```python
from build123d import *

# Parameters (mm, degrees)
F0_W          = 100.84
F0_H          = 99.31
F0_R          = 1.5
F0_R_2        = 2
F1_DEPTH      = 2
F3_W          = 15
F3_H          = 10
F3_W_2        = 41
F3_H_2        = 20.5
F4_DEPTH      = 13
F4_DEPTH_BACK = 2
F5_W          = 18
F5_H          = 35.5
F6_DEPTH      = 17
F8_W          = 8
F8_H          = 3
F9_DEPTH      = 2


with BuildPart() as f1:
    # F0 (on Top) → F1 (new body)
    with BuildSketch(Plane.XY):
        Rectangle(F0_W, F0_H)
        with Locations((-47.88, -46.865)):
            Circle(F0_R, mode=Mode.SUBTRACT)
        with Locations((-42.29, -44.825)):
            Circle(F0_R_2, mode=Mode.SUBTRACT)
        with Locations((-42.29, -36.445)):
            Circle(F0_R_2, mode=Mode.SUBTRACT)
        with Locations((-42.29, -24.765)):
            Circle(F0_R_2, mode=Mode.SUBTRACT)
        with Locations((-42.29, -16.635)):
            Circle(F0_R_2, mode=Mode.SUBTRACT)
        with Locations((-42.29, -4.955)):
            Circle(F0_R_2, mode=Mode.SUBTRACT)
        with Locations((42.29, -44.825)):
            Circle(F0_R_2, mode=Mode.SUBTRACT)
        with Locations((47.88, -46.865)):
            Circle(F0_R, mode=Mode.SUBTRACT)
        with Locations((42.29, -36.445)):
            Circle(F0_R_2, mode=Mode.SUBTRACT)
        with Locations((42.29, -24.765)):
            Circle(F0_R_2, mode=Mode.SUBTRACT)
        with Locations((42.29, -16.635)):
            Circle(F0_R_2, mode=Mode.SUBTRACT)
        with Locations((42.29, -4.955)):
            Circle(F0_R_2, mode=Mode.SUBTRACT)
        with Locations((-42.29, 3.175)):
            Circle(F0_R_2, mode=Mode.SUBTRACT)
        with Locations((-42.29, 14.855)):
            Circle(F0_R_2, mode=Mode.SUBTRACT)
        with Locations((-42.29, 22.985)):
            Circle(F0_R_2, mode=Mode.SUBTRACT)
        with Locations((-48.06, 25.525)):
            Circle(F0_R, mode=Mode.SUBTRACT)
        with Locations((42.29, 3.175)):
            Circle(F0_R_2, mode=Mode.SUBTRACT)
        with Locations((42.29, 14.855)):
            Circle(F0_R_2, mode=Mode.SUBTRACT)
        with Locations((42.29, 22.985)):
            Circle(F0_R_2, mode=Mode.SUBTRACT)
        with Locations((47.88, 25.275)):
            Circle(F0_R, mode=Mode.SUBTRACT)
    extrude(amount=F1_DEPTH)

    # F3 (on offset) → F4 (join, two sides)
    with BuildSketch(Plane.XY.offset(2)) as f4_sk:
        with Locations((-38.09, 54.655)):
            Rectangle(F3_W, F3_H)
        with Locations((23.92, 59.905)):
            Rectangle(F3_W_2, F3_H_2)
    extrude(amount=F4_DEPTH)
    extrude(f4_sk.sketch, amount=-F4_DEPTH_BACK)

    # F5 (on offset) → F6 (join)
    with BuildSketch(Plane.XY.offset(2)):
        with Locations((0, -31.905)):
            Rectangle(F5_W, F5_H)
    extrude(amount=F6_DEPTH)

    # F8 (on offset) → F9 (join)
    with BuildSketch(Plane.XZ.offset(49.655)):
        with Locations((0, 17.5)):
            Rectangle(F8_W, F8_H)
    extrude(amount=F9_DEPTH)


solid = f1.part
```
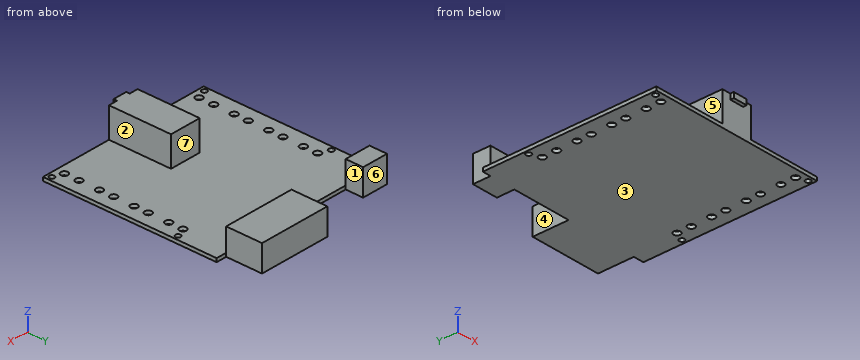
Geometry: final body of the model. Coordinates: model frame, mm. Face numbers are marked on the shaded views. A direction names the side the tool comes from. Give positions to 0.01 mm unless a question says otherwise; leave off trailing zeros. Loops run counter-clockwise (first coordinate to the right, second up) from the corner with the lowest first, then second, coordinate; pieces in that order, holes last. Notation, with made-up numbers: (-16, 26) -> (20, 26) arc R8 ccw to (20, 35) -> close; hole circle Ø10 at (-9.75, 57). An arc over 180 degrees is marked (long way). Use one line per item in the form item = value.
Item 1: Draft query along X for the marked faces 1, 2 and 3. Return one class per face: pulls with the +X half, pulls with the -X half, needs draft (parallel to the pull), parting line crosses it, or undercut.
A:
face_1 = undercut
face_2 = pulls with the +X half
face_3 = needs draft
Item 2: Access query for the marked faces 4, 5, 6 and 7. Directions: +Z, -Z, +X, -X, +Y, -Y. A direction counts if a zero-diameter tool reaches every point of the face in a straight line with its end or side. Return the directions, or none.
A:
face_4 = +Z, -Z, +Y
face_5 = +Z, -X, +Y, -Y
face_6 = +Z, -Z, -X, +Y
face_7 = +Z, +X, -X
Item 3: Section query A-A on z = 12.5. Output: boundary loops of the cut face in (x, y) (3 decimals), and give its area (3 significant figures).
A:
outline = (-45.59, 49.655) -> (-30.59, 49.655) -> (-30.59, 59.655) -> (-45.59, 59.655) -> close; (-9, -49.655) -> (9, -49.655) -> (9, -14.155) -> (-9, -14.155) -> close; (3.42, 49.655) -> (44.42, 49.655) -> (44.42, 70.155) -> (3.42, 70.155) -> close
area = 1,630 mm^2
Item 4: Line query: probe 1 along X at (y, z) = (56, 6.75); probe 2 along Y at (x, z) = (7.5, 5) (3 decimals); probe 3 along Z at (x, y) = (21, 15.5). Output: solid intervals per line, ascending.
A:
probe_1 = -45.59 to -30.59, 3.42 to 44.42
probe_2 = -49.655 to -14.155, 49.655 to 70.155
probe_3 = 0 to 2
Item 5: Section query C-C on x = -42.29. Give the number of separate pieces and of enclosed holes in the cut face, and give its area (3 significant figures).
A:
separate_pieces = 9
enclosed_holes = 0
area = 285 mm^2
Item 6: Section query D-D on y = 62. Output: boundary loops of the cut face in (x, z), and give its area (3 significant figures).
A:
outline = (3.42, 0) -> (44.42, 0) -> (44.42, 15) -> (3.42, 15) -> close
area = 615 mm^2
Item 7: Pin query (flat end, axial travel): P1, Ø6, axis at x = 22, y = 57.5, coming from the +Z side; P2, Ø5, axis at x = 8, y = 23.5, coming from the +Z side; P3, Ø2.5, axis at x = 42.29, y = -24.765, coming from the -Z side; P4, Ø2, axis at x = -9, z = 12, coming from the -Y side (3 decimals). Return the tip coordinate at first contact, or that it passes through.
A:
P1 = 15
P2 = 2
P3 = through
P4 = -49.655
Item 8: Section query B-B on x = 36. Output: boundary loops of the cut face in (y, z) (3 decimals), and give its area (3 significant figures).
A:
outline = (-49.655, 0) -> (70.155, 0) -> (70.155, 15) -> (49.655, 15) -> (49.655, 2) -> (-49.655, 2) -> close
area = 506 mm^2
